from build123d import *

# Parameters (mm, degrees)
BOSS_EXTRUDE1_DEPTH      = 50.9662557
BOSS_EXTRUDE1_DEPTH_BACK = 50.9662557
SKETCH1_R                = 4
CUT_EXTRUDE1_START       = -4.000000101
CUT_EXTRUDE1_OUTLINE_R   = 1.500000048
CUT_EXTRUDE1_DEPTH       = 8.000000202
CHAMFER1_SIZE            = 0.56


# Read off the part's stored shape, not the designer's step: Cut-Extrude1
with BuildPart() as part:
    # Sketch1 → Boss-Extrude1 (new, two sides: drawn at the far end of the back side and taken through both)
    with BuildSketch(Plane.XY.offset(-BOSS_EXTRUDE1_DEPTH_BACK)):
        Circle(SKETCH1_R)
    extrude(amount=BOSS_EXTRUDE1_DEPTH + BOSS_EXTRUDE1_DEPTH_BACK)

    # Cut-Extrude1 outline → Cut-Extrude1 (cut)
    with BuildSketch(Plane.YZ.offset(CUT_EXTRUDE1_START)):
        with Locations((0, -6.1352557)):
            Circle(CUT_EXTRUDE1_OUTLINE_R)
    extrude(amount=CUT_EXTRUDE1_DEPTH, mode=Mode.SUBTRACT)

    # Chamfer1
    chamfer1_edges = [part.edges().sort_by_distance(p)[0] for p in [
        (-4, 0, -50.9662557),
        (-4, 0, 50.9662557),
    ]]
    chamfer(chamfer1_edges, length=CHAMFER1_SIZE)


solid = part.part
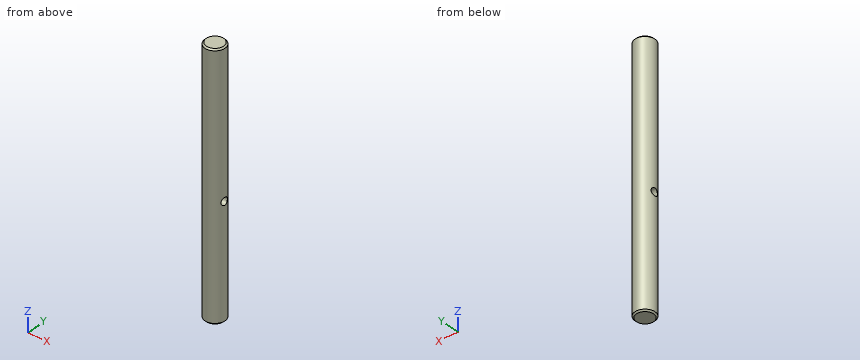
Could you check a few things on this model? Use its own coordinates, in mm. Coordinates: 2 decimals unless noted, no trailing zeros. Write each loop counter-clockwise with the first axis right and the second up, starting at its lowest first coordinate (ties: lowest second). Pieces come first, ordered by that corner, then holes. Notation, with made-up numbers: (16, -22) - (50, -22) arc R27 ccw to (50, 14) - close; hole circle Ø10 at (40.5, 43.5). An arc over 180 degrees is marked (long way). Put each result on its own line as item: value. Start each with the question number.
Q1. I want a section at A-A on y = 0. Write out the boundary of the cut face in (x, z), plus the area to 3 significant figures.
Q2. I'm going to push flat-ended pins straight in: P1, Ø2, axis at x = 2, z = 0, coming from the +Y side; P2, Ø1, axis at y = 3, z = 12, coming from the +X side; P3, Ø3, axis at x = -2.5, z = 26.5, coming from the -Y side; P4, Ø3, axis at x = -1.5, z = -32.5, coming from the +Y side. Where does each tip first touch, or does it pass through?
Q3. Please list where these lines run through material, in increasing order: L1, parallel to Z at x = -1.75, y = 0.25; L2, parallel to Z at x = -1, y = 0; L3, parallel to X at y = 2.5, z = 7.
Q4. I want a section at B-B on z = -38.5. Write out the boundary of the cut face in (x, y), plus the area to 3 significant figures.
Checks:
1. outline: (-4, -50.41) - (-3.44, -50.97) - (3.44, -50.97) - (4, -50.41) - (4, -7.64) - (-4, -7.64) - close; (-4, -4.64) - (4, -4.64) - (4, 50.41) - (3.44, 50.97) - (-3.44, 50.97) - (-4, 50.41) - close
1. area: 791 mm²
2. P1: y = 3.87
2. P2: x = 3.12
2. P3: y = -3.87
2. P4: y = 4
3. L1: -50.97 to -7.61, -4.66 to 50.97
3. L2: -50.97 to -7.64, -4.64 to 50.97
3. L3: -3.12 to 3.12
4. outline: circle Ø8 at (0, 0)
4. area: 50.3 mm²
